For this review, take the finished solid that the model builds, in its own axes (mm). Face numbers are marked on the shaded views. A direction names the side the tool comes from. Round coordinates to 2 decimals unless told otherwise and drop trailing zeros. Write each loop counter-clockwise with the first axis right and the second up, starting at its lowest first coordinate (ties: lowest second). Pieces come first, ordered by that corner, then holes. Notation, with made-up numbers: (81, 21) -> (94, 21) arc R23 ccw to (94, 29) -> close; hole circle Ø7 at (23, -23). An arc over 180 degrees is marked (long way). Answer in a Markdown table with one row per item. Add a question column.
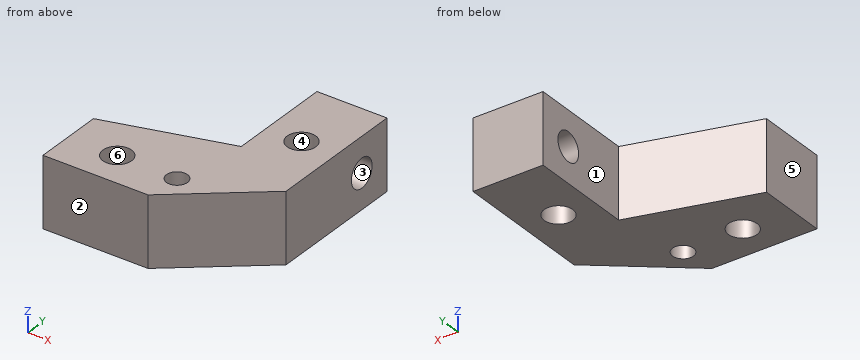
```python
from build123d import *

# Parameters (mm, degrees)
SKETCH_R     = 4.1
SKETCH_R_2   = 3
PAD_DEPTH    = 20
SKETCH001_R  = 4.1
POCKET_DEPTH = 55.001


with BuildPart() as part:
    # Sketch → Pad (new body)
    with BuildSketch(Plane.XY.offset(170)):
        Polygon((-30, 50), (-10, 50), (-10, 10), (-35, -10), (-65, -10), (-65, 10), (-30, 20), align=None)
        with Locations((-51, 0)):
            Circle(SKETCH_R, mode=Mode.SUBTRACT)
        with Locations((-33.8, -0.2)):
            Circle(SKETCH_R_2, mode=Mode.SUBTRACT)
        with Locations((-20, 30)):
            Circle(SKETCH_R, mode=Mode.SUBTRACT)
    extrude(amount=PAD_DEPTH)

    # Sketch001 → Pocket (cut, through all)
    with BuildSketch(Plane(origin=(-10, 0, 170), x_dir=(0, 1, 0), z_dir=(1, 0, 0))):
        with Locations((40, 10)):
            Circle(SKETCH001_R)
    extrude(amount=-POCKET_DEPTH, mode=Mode.SUBTRACT)


solid = part.part
```
1. We need section C-C (x = -20). Write out the cut boundary in (y, z).
2. We need section D-D (y = 29). Write out the cut boundary in (x, z), plus the area to 3 significant figures.
3. For L1, parallel to X at y = -1, z = 185.5; L2, parallel to X at y = 44.5, z = 185.5; L3, parallel to Y at x = -51, z = 178.25, list the stretches that pass through material, from the lowest coordinate up. Write a range as [from, to].
4. Clearance check with flat-ended pins moving along their axes: pin 1 Ø2 at (x, z) = (-58.5, 186.5) entering from +Y; pin 2 Ø4 at (x, z) = (-59, 175.5) entering from +Y; pin 3 Ø5 at (y, z) = (25, 181) entering from -X; pin 4 Ø3.5 at (x, y) = (-33.8, -0.2) entering from +Z. State where each tip first meets the part, or that it passes through.
5. We need section A-A (z = 180). Write out the cut boundary in (x, y), plus the area to 3 significant figures.
6. We need section B-B (x = -51). Write out the cut boundary in (y, z), plus the area to 3 significant figures.
7. The part is to be moulded in two halves that separate along X. For the marked faces 3, 4, 5 and 6, say which applies: pulls with the +X half, pulls with the -X half, needs draft (parallel to the pull), parting line crosses it, or undercut.
8. Tool access review of the marked faces 1 and 2: name each direction out of +Z, -Z, +X, -X, +Y, -Y from which nothing blocks a thin tool from reaching the whole face with its end or side.
Response:
| question | item | result |
|---|---|---|
| 1 | outline | (2, 170) -> (25.9, 170) -> (25.9, 190) -> (2, 190) -> close; (34.1, 170) -> (50, 170) -> (50, 190) -> (34.1, 190) -> close; hole circle Ø8.2 at (40, 180) |
| 2 | outline | (-30, 170) -> (-23.98, 170) -> (-23.98, 190) -> (-30, 190) -> close; (-16.02, 170) -> (-10, 170) -> (-10, 190) -> (-16.02, 190) -> close |
| 2 | area | 241 mm2 |
| 3 | L1 | [-65, -54.98], [-47.02, -36.69], [-30.91, -23.75] |
| 3 | L2 | [-30, -10] |
| 3 | L3 | [-10, -4.1], [4.1, 14] |
| 4 | pin 1 | y = 12.14 |
| 4 | pin 2 | y = 12.29 |
| 4 | pin 3 | x = -30 |
| 4 | pin 4 | through |
| 5 | outline | (-65, -10) -> (-35, -10) -> (-10, 10) -> (-10, 35.9) -> (-30, 35.9) -> (-30, 20) -> (-65, 10) -> close; (-30, 44.1) -> (-10, 44.1) -> (-10, 50) -> (-30, 50) -> close; hole circle Ø8.2 at (-51, 0); hole circle Ø6 at (-33.8, -0.2); hole circle Ø8.2 at (-20, 30) |
| 5 | area | 1,530 mm2 |
| 6 | outline | (-10, 170) -> (-4.1, 170) -> (-4.1, 190) -> (-10, 190) -> close; (4.1, 170) -> (14, 170) -> (14, 190) -> (4.1, 190) -> close |
| 6 | area | 316 mm2 |
| 7 | face 3 | needs draft |
| 7 | face 4 | undercut |
| 7 | face 5 | pulls with the -X half |
| 7 | face 6 | undercut |
| 8 | face 1 | +Z, -Z, -X, +Y |
| 8 | face 2 | +Z, -Z, +X, -X, -Y |
